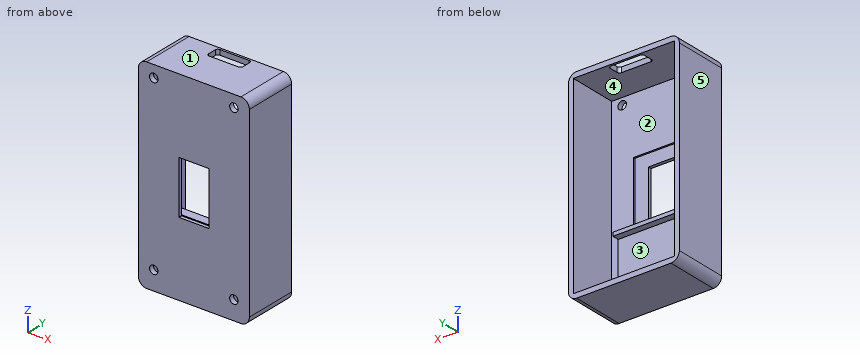
```python
from build123d import *

# Parameters (mm, degrees)
SKETCH1_W               = 33
SKETCH1_H               = 60
BOSS_EXTRUDE1_DEPTH     = 16
SHELL1_T                = -1.5
CUT_EXTRUDE2_DEPTH      = 10
SKETCH5_R               = 1.25
CUT_EXTRUDE3_DEPTH      = 1
CUT_EXTRUDE3_DEPTH_BACK = 3
SKETCH6_W               = 19.561169912
SKETCH6_H               = 0.704256658
BOSS_EXTRUDE2_DEPTH     = 18
SKETCH7_W               = 19.561169912
SKETCH7_H               = 1.086114883
BOSS_EXTRUDE3_DEPTH     = 2
SKETCH9_W               = 16.960059774
SKETCH9_H               = 23
CUT_EXTRUDE4_DEPTH      = 0.5
CUT_EXTRUDE6_REACH      = 18
SKETCH11_W              = 8.91696513
SKETCH11_H              = 15.868910044
FILLET1_R               = 2.5


with BuildPart() as part:
    # Sketch1 → Boss-Extrude1 (new body)
    with BuildSketch(Plane(origin=(0, 0, 0), x_dir=(1, 0, 0), z_dir=(0, 1, 0))):
        with Locations((16.989591658, -18.738797177)):
            Rectangle(SKETCH1_W, SKETCH1_H)
    extrude(amount=BOSS_EXTRUDE1_DEPTH)

    # Shell1
    shell1_openings = [part.faces().sort_by_distance(p)[0] for p in [
        (16.989591658, 16, 18.738797177),
    ]]
    offset(amount=SHELL1_T, openings=shell1_openings, kind=Kind.INTERSECTION)

    # Sketch4 → Cut-Extrude2 (cut)
    with BuildSketch(Plane.XY.offset(48.738797177)):
        with BuildLine():
            Line((12.619091925, 11.287469293), (21.360091391, 11.287469293))
            ThreePointArc((21.360091391, 11.287469293), (21.890421477, 11.507139207), (22.110091391, 12.037469293))
            Line((22.110091391, 12.037469293), (22.110091391, 14.61730298))
            ThreePointArc((22.110091391, 14.61730298), (21.890421477, 15.147633066), (21.360091391, 15.36730298))
            Line((21.360091391, 15.36730298), (12.619091925, 15.36730298))
            ThreePointArc((12.619091925, 15.36730298), (12.088761839, 15.147633066), (11.869091925, 14.61730298))
            Line((11.869091925, 14.61730298), (11.869091925, 12.037469293))
            ThreePointArc((11.869091925, 12.037469293), (12.088761839, 11.507139207), (12.619091925, 11.287469293))
        make_face()
    extrude(amount=-CUT_EXTRUDE2_DEPTH, mode=Mode.SUBTRACT)

    # Sketch5 → Cut-Extrude3 (cut, two sides)
    with BuildSketch(Plane.XZ) as cut_extrude3_sk:
        with Locations((28.889591658, 45.188797177)):
            Circle(SKETCH5_R)
        with Locations((5.089591658, 45.188797177)):
            Circle(SKETCH5_R)
        with Locations((28.889591658, -5.611202823)):
            Circle(SKETCH5_R)
        with Locations((5.089591658, -5.611202823)):
            Circle(SKETCH5_R)
    extrude(amount=CUT_EXTRUDE3_DEPTH, mode=Mode.SUBTRACT)
    extrude(cut_extrude3_sk.sketch, amount=-CUT_EXTRUDE3_DEPTH_BACK, mode=Mode.SUBTRACT)

    # Sketch6 → Boss-Extrude2 (add)
    with BuildSketch(Plane.XY.offset(-9.761202823)):
        with Locations((16.918287272, 5.415344609)):
            Rectangle(SKETCH6_W, SKETCH6_H)
    extrude(amount=BOSS_EXTRUDE2_DEPTH)

    # Sketch7 → Boss-Extrude3 (add)
    with BuildSketch(Plane(origin=(0, 5.767472938, 0), x_dir=(1, 0, 0), z_dir=(0, 1, 0))):
        with Locations((16.918287272, -7.695739736)):
            Rectangle(SKETCH7_W, SKETCH7_H)
    extrude(amount=BOSS_EXTRUDE3_DEPTH)

    # Sketch9 → Cut-Extrude4 (cut)
    with BuildSketch(Plane(origin=(0, 1.5, 0), x_dir=(1, 0, 0), z_dir=(0, 1, 0))):
        with Locations((16.989591658, -18.738797177)):
            Rectangle(SKETCH9_W, SKETCH9_H)
    extrude(amount=-CUT_EXTRUDE4_DEPTH, mode=Mode.SUBTRACT)

    # Sketch11 → Cut-Extrude6 (cut, up to next)
    with BuildSketch(Plane.XZ, mode=Mode.PRIVATE) as cut_extrude6_sk1:
        with Locations((17.046338664, 18.676425411)):
            Rectangle(SKETCH11_W, SKETCH11_H)
    cut_extrude6_tool1 = extrude(cut_extrude6_sk1.sketch, amount=-CUT_EXTRUDE6_REACH, mode=Mode.PRIVATE) & part.part
    add(cut_extrude6_tool1.solids().sort_by_distance((17.046339, 0, 18.676425))[0], mode=Mode.SUBTRACT)

    # Fillet1
    fillet1_edges = [part.edges().sort_by_distance(p)[0] for p in [
        (0.489591658, 8, -11.261202823),
        (33.489591658, 8, -11.261202823),
        (33.489591658, 8, 48.738797177),
        (0.489591658, 8, 48.738797177),
    ]]
    fillet(fillet1_edges, radius=FILLET1_R)


solid = part.part
```
Read the model definition and answer for the solid it produces. Units are mm, in the model's axes. Face numbers are marked on the shaded views. A direction names the side the tool comes from. Give positions to 0.01 mm unless a question says otherwise; leave off trailing zeros. Write each loop counter-clockwise with the first axis right and the second up, starting at its lowest first coordinate (ties: lowest second). Pieces come first, ordered by that corner, then holes. Notation, with made-up numbers: (-14, 9.25) -> (6, 9.25) arc R19 ccw to (6, 41.25) -> close; hole circle Ø2 at (-0.5, 47). An arc over 180 degrees is marked (long way). Answer as a JSON object with one key per item and string values.
1) Flat-ended cylindrical pins translate along their axes: pin 1 Ø2 at (x, z) = (28.89, -5.61) entering from -Y; pin 2 Ø5 at (x, z) = (14, 23.5) entering from +Y; pin 3 Ø13.5 at (x, z) = (19, 0) entering from +Y; pin 4 Ø3 at (x, z) = (5.09, -5.61) entering from +Y. Find the tip coordinate at first contact, or state that the pin passes through.
Findings below:
{"pin 1": "passes through", "pin 2": "stops at y = 1", "pin 3": "stops at y = 5.77", "pin 4": "stops at y = 1.5"}
2) Straight lines are drawn through the part: probe 1 along Z at (x, y) = (28.5, 5.25); probe 2 along X at (y, z) = (13, 34.5); probe 3 along Y at (x, z) = (21, 0.5). For each, find the intervals that lie inside material, in ascending order. Write a range as from..to.
Findings below:
{"probe 1": "z = -11.26..-9.76, 47.24..48.74", "probe 2": "x = 0.49..1.99, 31.99..33.49", "probe 3": "y = 0..1.5, 5.06..5.77"}
3) Section A-A on x = 15.5 is taken. Write down the section's boundary in (y, z), then the cut area to 3 significant figures.
Findings below:
{"outline": "(0, -11.26) -> (16, -11.26) -> (16, -9.76) -> (5.77, -9.76) -> (5.77, 7.15) -> (7.77, 7.15) -> (7.77, 8.24) -> (5.06, 8.24) -> (5.06, -9.76) -> (1.5, -9.76) -> (1.5, 7.24) -> (1, 7.24) -> (1, 10.74) -> (0, 10.74) -> close; (0, 26.61) -> (1, 26.61) -> (1, 30.24) -> (1.5, 30.24) -> (1.5, 47.24) -> (11.29, 47.24) -> (11.29, 48.74) -> (0, 48.74) -> close; (15.37, 47.24) -> (16, 47.24) -> (16, 48.74) -> (15.37, 48.74) -> close", "area": "115 mm^2"}
4) Section C-C on y = 8.75 is taken. Write down the section's boundary in (x, z).
Findings below:
{"outline": "(0.49, -8.76) arc R2.5 ccw to (2.99, -11.26) -> (30.99, -11.26) arc R2.5 ccw to (33.49, -8.76) -> (33.49, 46.24) arc R2.5 ccw to (30.99, 48.74) -> (2.99, 48.74) arc R2.5 ccw to (0.49, 46.24) -> close; hole (1.99, -9.76) -> (31.99, -9.76) -> (31.99, 47.24) -> (1.99, 47.24) -> close"}
5) For a pull along Y with two mould halves and no side action, classify the marked faces 1, 2 and 3 as pulls with the +Y half, pulls with the -Y half, needs draft (parallel to the pull), parting line crosses it, or undercut.
Findings below:
{"face 1": "needs draft", "face 2": "undercut", "face 3": "pulls with the +Y half"}
6) Section D-D on x = 10.5 is taken. Write down the section's boundary in (y, z), then the cut area to 3 significant figures.
Findings below:
{"outline": "(0, -11.26) -> (16, -11.26) -> (16, -9.76) -> (5.77, -9.76) -> (5.77, 7.15) -> (7.77, 7.15) -> (7.77, 8.24) -> (5.06, 8.24) -> (5.06, -9.76) -> (1.5, -9.76) -> (1.5, 7.24) -> (1, 7.24) -> (1, 30.24) -> (1.5, 30.24) -> (1.5, 47.24) -> (16, 47.24) -> (16, 48.74) -> (0, 48.74) -> close", "area": "137 mm^2"}
7) Section B-B on z = 17 is taken. Write down the section's boundary in (x, y).
Findings below:
{"outline": "(0.49, 0) -> (12.59, 0) -> (12.59, 1) -> (8.51, 1) -> (8.51, 1.5) -> (1.99, 1.5) -> (1.99, 16) -> (0.49, 16) -> close; (21.5, 0) -> (33.49, 0) -> (33.49, 16) -> (31.99, 16) -> (31.99, 1.5) -> (25.47, 1.5) -> (25.47, 1) -> (21.5, 1) -> close"}
8) A tool of negligible diameter and unlimited length cuts with its end or side. For the marked faces 4 and 5, from which of +Z, -Z, +X, -X, +Y, -Y can it reach the whole face along a straight path? Write none if from no direction.
Findings below:
{"face 4": "+Y", "face 5": "+Z, -Z, -X, +Y, -Y"}
